Autodesk Inventor part; units mm, degrees
ref_plane "YZ Plane" through (0, 0, 0) normal (1, 0, 0) x (0, 1, 0)
ref_plane "XZ Plane" through (0, 0, 0) normal (0, 1, 0) x (-1, 0, 0)
ref_plane "XY Plane" through (0, 0, 0) normal (0, 0, 1) x (1, 0, 0)
sketch "Sketch1" plane through (0, 0, 0) normal (0, 1, 0) x (-1, 0, 0)
  line L0 (0, 0) -> (42.3, 0)
  line L1 (42.3, 0) -> (42.3, -42.3)
  line L2 (42.3, -42.3) -> (0, -42.3)
  line L3 (0, -42.3) -> (0, 0)
  circle A0 centre (21.15, -21.15) radius 5.15
  circle A1 centre (29.15, -21.15) radius 1.8
  circle A2 centre (21.15, -21.15) radius 8
  circle A3 centre (21.15, -13.15) radius 1.8
  circle A4 centre (13.15, -21.15) radius 1.8
  circle A5 centre (21.15, -29.15) radius 1.8
  point P0 (0, -21.15)
  point P1 (21.15, -42.3)
  dimension "d4" = 16
  dimension "d0" = 42.3
  dimension "d2" = 10.3
  dimension "d3" = 3.6
  dimension "d7" = 360
extrude "Extrusion1" add sketch "Sketch1" along normal blind 10 contours L0 L1 L2 L3 | A1 A2 A5 A4 A3
sketch "Sketch2" plane through (0, 10, 0) normal (0, 1, 0) x (1, 0, 0)
  line L0 (-42.3, 0) -> (0, 0) construction
  circle A0 centre (-13.15, 21.15) radius 1.8 construction
  circle A1 centre (-29.15, 21.15) radius 1.8 construction
  line L1 (-42.3, 0) -> (0, 0) construction
  line L2 (-16.25, 0) -> (-16.25, -3.81)
  line L3 (-16.25, -3.81) -> (-26.05, -3.81)
  line L4 (-26.05, -3.81) -> (-26.05, 0)
  line L5 (-26.05, 0) -> (-16.25, 0)
  line L6 (-13.15, 21.15) -> (-29.15, 21.15)
  line L7 (-42.3, 42.3) -> (0, 42.3) construction
  line L8 (-42.3, 42.3) -> (0, 42.3) construction
  line L9 (-16.25, 42.3) -> (-16.25, 46.11)
  line L10 (-16.25, 46.11) -> (-26.05, 46.11)
  line L11 (-26.05, 46.11) -> (-26.05, 42.3)
  line L12 (-26.05, 42.3) -> (-16.25, 42.3)
  line L13 (-16.25, 46.11) -> (-16.25, 46.31)
  line L14 (-16.25, 46.31) -> (-11.424, 46.31)
  line L15 (-11.424, 46.31) -> (-11.424, 51.136)
  line L16 (-26.05, 46.11) -> (-26.05, 46.31)
  line L17 (-26.05, 46.31) -> (-30.876, 46.31)
  line L18 (-30.876, 46.31) -> (-30.876, 51.136)
  line L19 (-30.876, 51.136) -> (-11.424, 51.136)
  line L20 (-16.25, -3.81) -> (-16.25, -4.01)
  line L21 (-16.25, -4.01) -> (-11.424, -4.01)
  line L22 (-11.424, -4.01) -> (-11.424, -8.836)
  line L23 (-26.05, -3.81) -> (-26.05, -4.01)
  line L24 (-26.05, -4.01) -> (-30.876, -4.01)
  line L25 (-30.876, -4.01) -> (-30.876, -8.836)
  line L26 (-30.876, -8.836) -> (-11.424, -8.836)
  point P0 (-21.15, -3.81)
  point P1 (-21.15, 0)
  point P2 (-21.15, 46.11)
  point P3 (-21.15, 42.3)
  dimension "d11" = 3.81
  dimension "d12" = 9.8
  dimension "d28" = 0.2
  dimension "d29" = 4.826
  dimension "d30" = 4.826
  dimension "d31" = 0.2
  dimension "d32" = 4.826
  dimension "d33" = 4.826
extrude "Extrusion2" add sketch "Sketch2" against normal blind 10
sketch "Sketch3" plane through (0, 0, 0) normal (0, -1, 0) x (1, 0, 0)
  circle A0 centre (-13.15, -21.15) radius 1.8 construction
  circle A1 centre (-29.15, -21.15) radius 1.8 construction
  line L0 (-13.15, -21.15) -> (-29.15, -21.15)
  line L1 (-16.25, 0) -> (-16.25, 4.01) construction
  line L2 (-11.424, 4.01) -> (-11.424, 8.836) construction
  line L3 (-30.876, 8.836) -> (-30.876, 4.01) construction
  line L4 (-30.876, 4.01) -> (-26.05, 4.01) construction
  line L5 (-26.05, 4.01) -> (-26.05, 0) construction
  line L6 (-16.25, 4.01) -> (-11.424, 4.01)
  line L7 (-11.424, 4.01) -> (-11.424, 8.836)
  line L8 (-11.424, 8.836) -> (-30.876, 8.836)
  line L9 (-30.876, 8.836) -> (-30.876, 4.01)
  line L10 (-30.876, 4.01) -> (-26.05, 4.01)
  line L11 (-26.05, 4.01) -> (-26.05, 2.105)
  line L12 (-26.05, 2.105) -> (-16.25, 2.005)
  line L13 (-16.25, 4.01) -> (-16.25, 2.005)
  line L14 (-16.25, -42.3) -> (-16.25, -46.31) construction
  line L15 (-16.25, -46.31) -> (-11.424, -46.31) construction
  line L16 (-11.424, -46.31) -> (-11.424, -51.136) construction
  line L17 (-11.424, -51.136) -> (-30.876, -51.136) construction
  line L18 (-30.876, -51.136) -> (-30.876, -46.31) construction
  line L19 (-30.876, -46.31) -> (-26.05, -46.31) construction
  line L20 (-26.05, -46.31) -> (-26.05, -42.3) construction
  line L21 (-16.25, -46.31) -> (-11.424, -46.31)
  line L22 (-11.424, -46.31) -> (-11.424, -51.136)
  line L23 (-11.424, -51.136) -> (-30.876, -51.136)
  line L24 (-30.876, -51.136) -> (-30.876, -46.31)
  line L25 (-30.876, -46.31) -> (-26.05, -46.31)
  line L26 (-26.05, -46.31) -> (-26.05, -44.405)
  line L27 (-26.05, -44.405) -> (-16.25, -44.305)
  line L28 (-16.25, -46.31) -> (-16.25, -44.305)
  dimension "d34" = 1.905
extrude "Extrusion3" add sketch "Sketch3" along normal blind 91.6
sketch "Sketch4" plane through (0, 10, 0) normal (0, 1, 0) x (1, 0, 0)
  line L0 (-42.3, 0) -> (-135.01, 0)
  line L1 (-135.01, 0) -> (-135.01, 42.3)
  line L2 (-135.01, 42.3) -> (-42.3, 42.3)
  line L3 (-42.3, 0) -> (-42.3, 42.3)
  dimension "d17" = 92.71
extrude "Extrusion4" add sketch "Sketch4" against normal blind 10
sketch "Sketch5" plane through (0, 0, 0) normal (0, -1, 0) x (1, 0, 0)
  line L0 (-135.01, 0) -> (-135.01, -42.3) construction
  line L1 (-122.31, -36.0725) -> (-51.19, -36.0725)
  line L2 (-51.19, -36.0725) -> (-51.19, -6.2275)
  line L3 (-51.19, -6.2275) -> (-122.31, -6.2275)
  line L4 (-122.31, -6.2275) -> (-122.31, -36.0725)
  point P0 (-135.01, -7.62)
  point P1 (-135.01, -34.68)
  point P2 (-122.31, -21.15)
  point P3 (-135.01, -21.15)
  dimension "d35" = 71.12
  dimension "d36" = 29.845
  dimension "d37" = 12.7
extrude "Extrusion5" cut sketch "Sketch5" against normal blind 5
sketch "Sketch6" plane through (0, 10, 0) normal (0, 1, 0) x (1, 0, 0)
  line L0 (-135.01, 0) -> (-26.05, 0) construction
  line L1 (-30.876, -8.836) -> (-11.424, -8.836) construction
  line L2 (0, 0) -> (0, 42.3) construction
  line L3 (-11.424, 51.136) -> (-30.876, 51.136) construction
  line L4 (-30.876, 51.136) -> (-30.876, 46.31) construction
  line L5 (-26.05, 42.3) -> (-135.01, 42.3) construction
  line L6 (-135.01, 42.3) -> (-135.01, 0) construction
  circle A0 centre (-21.15, 21.15) radius 5.15 construction
  circle A1 centre (-21.15, 21.15) radius 11.43
  line L7 (0, 42.3) -> (0, 0)
  line L8 (0, 0) -> (-11.424, -8.836)
  line L9 (0, 42.3) -> (-11.424, 51.136)
  line L10 (-11.424, 51.136) -> (-30.876, 51.136)
  line L11 (-30.876, 51.136) -> (-30.876, 42.3)
  line L12 (-11.424, -8.836) -> (-30.876, -8.836)
  line L13 (-30.876, -8.836) -> (-30.876, 0)
  line L14 (-30.876, 0) -> (-135.01, 0)
  line L15 (-135.01, 0) -> (-135.01, 42.3)
  line L16 (-135.01, 42.3) -> (-30.876, 42.3)
  dimension "d40" = 22.86
extrude "Extrusion6" [suppressed]
chamfer "Chamfer3" [suppressed]
chamfer "Chamfer4" [suppressed]
sketch "Sketch7" plane through (-26.05, 10, -42.3) normal (0, 0, -1) x (-1, 0, 0)
  line L0 (5.08, 0) -> (5.08, 39.5) construction
  line L1 (0, -10) -> (108.96, -10) construction
  circle A0 centre (68.58, 2.7) radius 3.175
  circle A1 centre (55.88, 2.7) radius 3.175
  circle A2 centre (43.18, 2.7) radius 3.175
  circle A3 centre (30.48, 2.7) radius 3.175
  circle A4 centre (17.78, 2.7) radius 3.175
  circle A5 centre (62.23, 15.4) radius 3.175
  circle A6 centre (49.53, 15.4) radius 3.175
  circle A7 centre (36.83, 15.4) radius 3.175
  circle A8 centre (24.13, 15.4) radius 3.175
  circle A9 centre (11.43, 15.4) radius 3.175
  point P0 (101.34, -10)
  point P1 (-26.05, -10)
  dimension "d49" = 6.35
  dimension "d50" = 12.7
  dimension "d51" = 12.7
  dimension "d52" = 12.7
  dimension "d53" = 12.7
  dimension "d54" = 12.7
  dimension "d55" = 12.7
  dimension "d56" = 6.35
  dimension "d57" = 12.7
  dimension "d58" = 12.7
  dimension "d59" = 12.7
  dimension "d60" = 12.7
  dimension "d61" = 6.35
  dimension "d62" = 12.7
extrude "Extrusion7" [suppressed]
properties part number "ClawGrip"
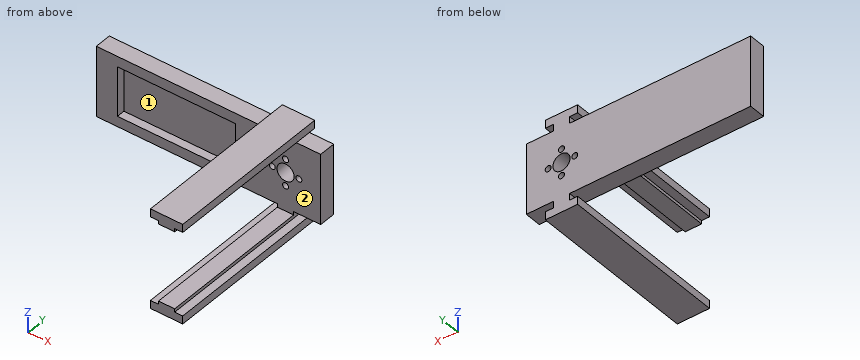
Work out the finished part from the listing and answer in its coordinate system (mm). Face numbers are marked on the shaded views. Coordinates: 2 decimals unless noted, no trailing zeros. Loops run counter-clockwise (first coordinate to the right, second up) from the corner with the lowest first, then second, coordinate; pieces in that order, holes last.
1) For a pull along X with two mould halves and no side action, classify the marked faces 1 and 2 as +X half, -X half, draft (parallel to the pull), parting line (faces both ways), or undercut.
Results:
face 1: undercut
face 2: draft
2) Consider probe 1 along X at (y, z) = (3.5, -29.15); probe 2 along Z at (x, y) = (-13, 3); probe 3 along Z at (x, y) = (-21.15, 5.5). Determine where each line is inside the solid, lowest interval first.
Results:
probe 1: x = -135.01 to -122.31, -51.19 to -22.95, -19.35 to 0
probe 2: z = -51.14 to -46.31, -42.3 to -22.94, -19.36 to 0, 4.01 to 8.84
probe 3: z = -51.14 to -30.95, -27.35 to -26.3, -16 to -14.95, -11.35 to 8.84
3) Section D-D (z = -8) is taken. Give the vertices of the cut face in (x, y), plus the area to 4 significant figures.
Results:
outline: (-135.01, 0) - (-122.31, 0) - (-122.31, 5) - (-51.19, 5) - (-51.19, 0) - (0, 0) - (0, 10) - (-135.01, 10) - close
area: 994.5 mm2
4) Section B-B (z = -29.15) is taken. Give the vertices of the cut face in (x, y).
Results:
outline: (-135.01, 0) - (-122.31, 0) - (-122.31, 5) - (-51.19, 5) - (-51.19, 0) - (-22.95, 0) - (-22.95, 10) - (-135.01, 10) - close; (-19.35, 0) - (0, 0) - (0, 10) - (-19.35, 10) - close
5) Section A-A (y = -72) is taken. Give the vertices of the cut face in (x, z) (3 decimals).
Results:
outline: (-30.876, -51.136) - (-11.424, -51.136) - (-11.424, -46.31) - (-16.25, -46.31) - (-16.25, -44.305) - (-26.05, -44.405) - (-26.05, -46.31) - (-30.876, -46.31) - close; (-30.876, 4.01) - (-26.05, 4.01) - (-26.05, 2.105) - (-16.25, 2.005) - (-16.25, 4.01) - (-11.424, 4.01) - (-11.424, 8.836) - (-30.876, 8.836) - close
6) Flat-ended cylindrical pins translate along their axes: pin 1 (5.5 mm diameter, centred on x = -88, y = 1.5, fed in from +Z); pin 2 (1.4 mm diameter, centred on y = -60.5, z = -49, fed in from -X); pin 3 (1.2 mm diameter, centred on y = -26, z = 1.5, fed in from +X); pin 4 (12 mm diameter, centred on y = -4.5, z = -40, fed in from -X). Find the tip coordinate at first contact, or state that the pin passes through.
Results:
pin 1: stops at z = 0
pin 2: stops at x = -30.88
pin 3: stops at x = -16.25
pin 4: stops at x = -135.01
7) Section C-C (x = -13.15) is taken. Give the vertices of the cut face in (y, z), plus the area to 3 significant figures.
Results:
outline: (-91.6, -51.14) - (10, -51.14) - (10, -46.31) - (-91.6, -46.31) - close; (-91.6, 4.01) - (10, 4.01) - (10, 8.84) - (-91.6, 8.84) - close; (0, -42.3) - (10, -42.3) - (10, -22.95) - (0, -22.95) - close; (0, -19.35) - (10, -19.35) - (10, 0) - (0, 0) - close
area: 1,370 mm2
